The model under review builds one solid part; all positions refer to its coordinate system, in mm. Give positions to 0.01 mm unless a question says otherwise; leave off trailing zeros. Order: outer loops, then holes, each group sorted by start corner. A loop starts at its lowest first (then second) coordinate and runs counter-clockwise, first axis right, second up.
Autodesk Inventor part; units mm, degrees
ref_plane "YZ Plane" through (0, 0, 0) normal (1, 0, 0) x (0, 1, 0)
ref_plane "XZ Plane" through (0, 0, 0) normal (0, 1, 0) x (-1, 0, 0)
ref_plane "XY Plane" through (0, 0, 0) normal (0, 0, 1) x (1, 0, 0)
sketch "Sketch1" plane through (0, 0, 0) normal (1, 0, 0) x (0, 1, 0)
  line L0 (3.3442, 266.7) -> (6.35, 266.7)
  line L1 (6.35, 266.7) -> (6.35, 254)
  line L2 (6.35, 254) -> (0, 254)
  line L3 (0, 254) -> (0, 0)
  line L4 (0, 0) -> (-12.7, 0) construction
  line L5 (-12.7, 0) -> (-12.7, 190.5)
  line L6 (-12.7, 215.9) -> (-12.7, 266.7)
  line L7 (3.3442, 266.7) -> (-12.7, 266.7)
  line L8 (3.3442, -266.7) -> (6.35, -266.7)
  line L9 (6.35, -266.7) -> (6.35, -254)
  line L10 (6.35, -254) -> (0, -254)
  line L11 (0, -254) -> (0, 0)
  line L12 (-12.7, 0) -> (-12.7, -190.5)
  line L13 (-12.7, -215.9) -> (-12.7, -266.7)
  line L14 (3.3442, -266.7) -> (-12.7, -266.7)
  line L15 (-12.7, 215.9) -> (-12.7, 190.5)
  line L16 (-12.7, -190.5) -> (-12.7, -215.9)
  dimension "d1" = 12.7
  dimension "d3" = 6.35
  dimension "d4" = 254
  dimension "d5" = 12.7
extrude "Extrusion1" add sketch "Sketch1" along normal blind 12.7
sketch "Sketch4" plane through (12.7, 0, 0) normal (1, 0, 0) x (0, 0, -1)
  circle A0 centre (-215.9, -6.35) radius 2.921
  line L0 (-266.7, 6.35) -> (-266.7, -12.7)
  line L1 (254, 0) -> (-254, 0)
  point P0 (0, 0)
  dimension "d32" = 5.842
  dimension "d33" = 50.8
  dimension "d34" = 6.35
hole "Hole3" at (12.7, -6.35, 215.9) direction (-1, 0, 0) diameter 5.842 end through all
mirror "Mirror3" about plane through (0, 0, 0) normal (0, 0, 1) of "Hole3"
properties part number "Support GuideRail"
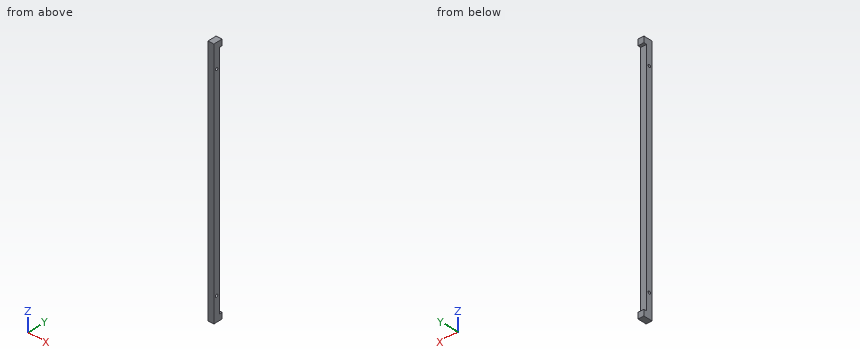
Item 1: Take a section at C-C (z = -71). Give the boundary of the cut face in (x, y), and give its area (3 significant figures).
Values found:
outline: (0, -12.7) - (12.7, -12.7) - (12.7, 0) - (0, 0) - close
area: 161 mm2
Item 2: Clearance check with flat-ended pins moving along their axes: pin 1 Ø6.5 at (x, z) = (3.5, -117) entering from +Y; pin 2 Ø4.5 at (y, z) = (-6.35, -215.9) entering from -X. State where each tip first meets the part, or that it passes through.
Values found:
pin 1: stops at y = 0
pin 2: passes through
Item 3: For line 1 (Z direction, x = 6.5, y = -6.35); line 2 (Y direction, x = 5.5, z = -215.9); line 3 (Z direction, x = 5.5, y = 3.5), list the stretches that pass through material, from the lowest coordinate up.
Values found:
line 1: z = -266.7 to -218.82, -212.98 to 212.98, 218.82 to 266.7
line 2: y = -12.7 to -9.27, -3.43 to 0
line 3: z = -266.7 to -254, 254 to 266.7
Item 4: Take a section at B-B (x = 8.5). Give the boundary of the cut face in (y, z).
Values found:
outline: (-12.7, -266.7) - (6.35, -266.7) - (6.35, -254) - (0, -254) - (0, 254) - (6.35, 254) - (6.35, 266.7) - (-12.7, 266.7) - close; hole circle Ø5.84 at (-6.35, -215.9); hole circle Ø5.84 at (-6.35, 215.9)
Item 5: Take a section at A-A (y = -6.35). Give the boundary of the cut face in (x, z), and give its area (3 significant figures).
Values found:
outline: (0, -266.7) - (12.7, -266.7) - (12.7, -218.82) - (0, -218.82) - close; (0, -212.98) - (12.7, -212.98) - (12.7, 212.98) - (0, 212.98) - close; (0, 218.82) - (12.7, 218.82) - (12.7, 266.7) - (0, 266.7) - close
area: 6,630 mm2
